Part print with two shaded views. Sizes in mm from the minimum x, y, z corner. A direction names the side the tool comes from. Give positions to 0.01 mm unless a question says otherwise; leave off trailing zeros. Order: outer loops, then holes, each group sorted by start corner. A loop starts at its lowest first (then second) coordinate and runs counter-clockwise, first axis right, second up. Notation, with made-up numbers: (49, 77) -> (55, 77) arc R28 ccw to (55, 115) -> close; hole circle Ø4 at (8.25, 83). An arc over 180 degrees is marked (long way). Answer in a Markdown table with one row per item. Add a question column.
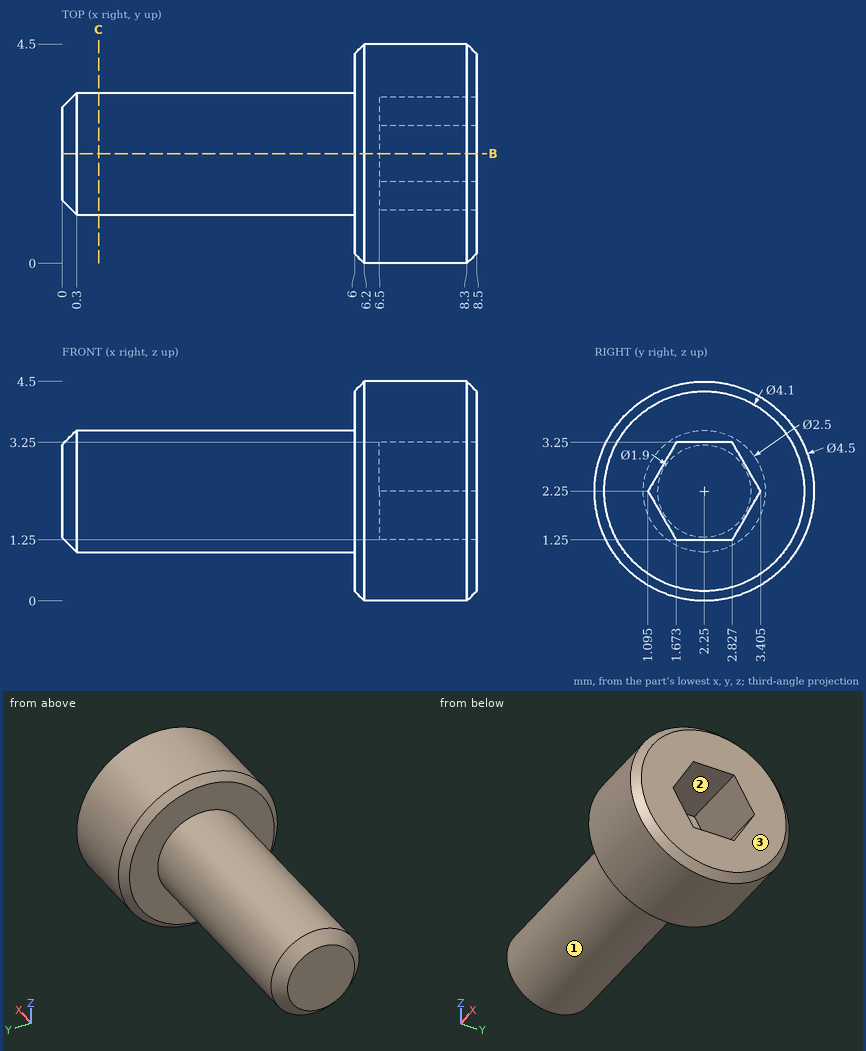
Item 1: Saw through at B-B on y = 2.25. List the corners of the cut face in (x, z), plus the area to 3 significant figures.
Item 2: Which spindle directions (+Z, -Z, +X, -X, +Y, -Y) get a long thin tool onto all of the face, cutting with end or side? Do the marked faces 1, 2 and 3. Say none if no direction does.
Item 3: Pin check, flat tip, straight feed: pin 1 Ø1 at (x, y) = (5, 1.5) entering from +Z (1 decimal). Stop position of the tip, or through.
Item 4: Saw through at C-C on x = 0.75. List the corners of the cut face in (y, z).
Item 5: Wall check: line 1 (X direction, y = 2.1, z = 0.6); line 2 (X direction, y = 2.05, z = 2.8); line 3 (Z direction, x = 7.5, y = 1.2). Give the ranges that are in metal, low to high.
Evaluation:
| question | item | result |
|---|---|---|
| 1 | outline | (0, 1.3) -> (0.3, 1) -> (6, 1) -> (6, 0.2) -> (6.2, 0) -> (8.3, 0) -> (8.5, 0.2) -> (8.5, 1.25) -> (6.5, 1.25) -> (6.5, 3.25) -> (8.5, 3.25) -> (8.5, 4.3) -> (8.3, 4.5) -> (6.2, 4.5) -> (6, 4.3) -> (6, 3.5) -> (0.3, 3.5) -> (0, 3.2) -> close |
| 1 | area | 22.1 mm2 |
| 2 | face 1 | -X |
| 2 | face 2 | +X |
| 2 | face 3 | +Z, -Z, +X, +Y, -Y |
| 3 | pin 1 | stops at z = 3.5 |
| 4 | outline | circle Ø2.5 at (2.25, 2.25) |
| 5 | line 1 | x = 6 to 8.5 |
| 5 | line 2 | x = 0 to 6.5 |
| 5 | line 3 | z = 0.26 to 2.07, 2.43 to 4.24 |
